Part model, mm, in its own coordinate system. Give positions to 0.01 mm unless a question says otherwise; leave off trailing zeros. Loops run counter-clockwise (first coordinate to the right, second up) from the corner with the lowest first, then second, coordinate; pieces in that order, holes last. Notation, with made-up numbers: (9.25, 36.25) -> (24.25, 36.25) arc R14 ccw to (24.25, 61.25) -> close; hole circle Ø2 at (81.25, -17). An arc over 180 degrees is marked (long way). Write item = value, one per line.
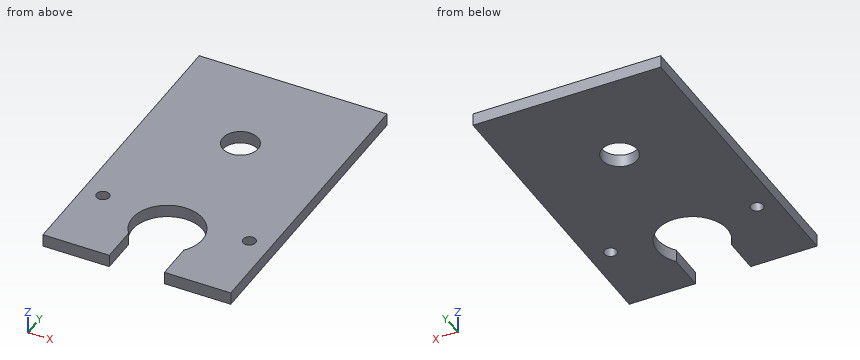
from build123d import *

# Parameters (mm, degrees)
ESQUISSE1_W             = 150
ESQUISSE1_H             = 240
BASE_EXTRUSION_DEPTH    = 10
ENL_V_MAT_EXTRU_1_DEPTH = 10
ESQUISSE3_R             = 14.142135624
ENL_V_MAT_EXTRU_2_DEPTH = 10
ESQUISSE4_R             = 5
ENL_V_MAT_EXTRU_3_DEPTH = 284.19604517


with BuildPart() as part:
    # Esquisse1 → Base-Extrusion (new body)
    with BuildSketch(Plane.XY):
        with Locations((75, 120)):
            Rectangle(ESQUISSE1_W, ESQUISSE1_H)
    extrude(amount=BASE_EXTRUSION_DEPTH)

    # Esquisse2 → Enlèv. mat.-Extru.1 (cut)
    with BuildSketch(Plane.XY.offset(10)):
        with BuildLine():
            Line((53, 0), (97, 0))
            Line((97, 0), (97, 29.679491924))
            ThreePointArc((97, 29.679491924), (75, 75), (53, 29.679491924))
            Line((53, 29.679491924), (53, 0))
        make_face()
    extrude(amount=-ENL_V_MAT_EXTRU_1_DEPTH, mode=Mode.SUBTRACT)

    # Esquisse3 → Enlèv. mat.-Extru.2 (cut)
    with BuildSketch(Plane.XY.offset(10)):
        with Locations((74, 161)):
            Circle(ESQUISSE3_R)
    extrude(amount=-ENL_V_MAT_EXTRU_2_DEPTH, mode=Mode.SUBTRACT)

    # Esquisse4 → Enlèv. mat.-Extru.3 (cut, through all)
    with BuildSketch(Plane(origin=(0, 0, 0), x_dir=(-1, 0, 0), z_dir=(0, 0, -1))):
        with Locations((-16.142927736, 61)):
            Circle(ESQUISSE4_R)
        with Locations((-133.142927736, 61)):
            Circle(ESQUISSE4_R)
    extrude(amount=-ENL_V_MAT_EXTRU_3_DEPTH, mode=Mode.SUBTRACT)


solid = part.part
1) Slice it at C-C, the plane x = 73. List the corners of the cut face in (y, z).
Resolved:
outline = (74.93, 0) -> (146.89, 0) -> (146.89, 10) -> (74.93, 10) -> close; (175.11, 0) -> (240, 0) -> (240, 10) -> (175.11, 10) -> close
2) Slice it at A-A, the plane y = 47. List the corners of the cut face in (x, z), and give its area (3 significant figures).
Resolved:
outline = (0, 0) -> (47, 0) -> (47, 10) -> (0, 10) -> close; (103, 0) -> (150, 0) -> (150, 10) -> (103, 10) -> close
area = 940 mm²
3) Slice it at B-B, the plane z = 4. List the corners of the cut face in (x, y).
Resolved:
outline = (0, 0) -> (53, 0) -> (53, 29.68) arc R28 cw (long way) to (97, 29.68) -> (97, 0) -> (150, 0) -> (150, 240) -> (0, 240) -> close; hole circle Ø10 at (16.14, 61); hole circle Ø28.28 at (74, 161); hole circle Ø10 at (133.14, 61)
4) Drill centre lines: line 1 along X through (y, z) = (47, 6.5); line 2 along X through (y, z) = (155.5, 9.25); line 3 along Y through (x, z) = (14, 7.5). Where is each one in solid material? Low to high. Write a range as [from, to].
Resolved:
line_1 = [0, 47], [103, 150]
line_2 = [0, 60.97], [87.03, 150]
line_3 = [0, 56.48], [65.52, 240]
